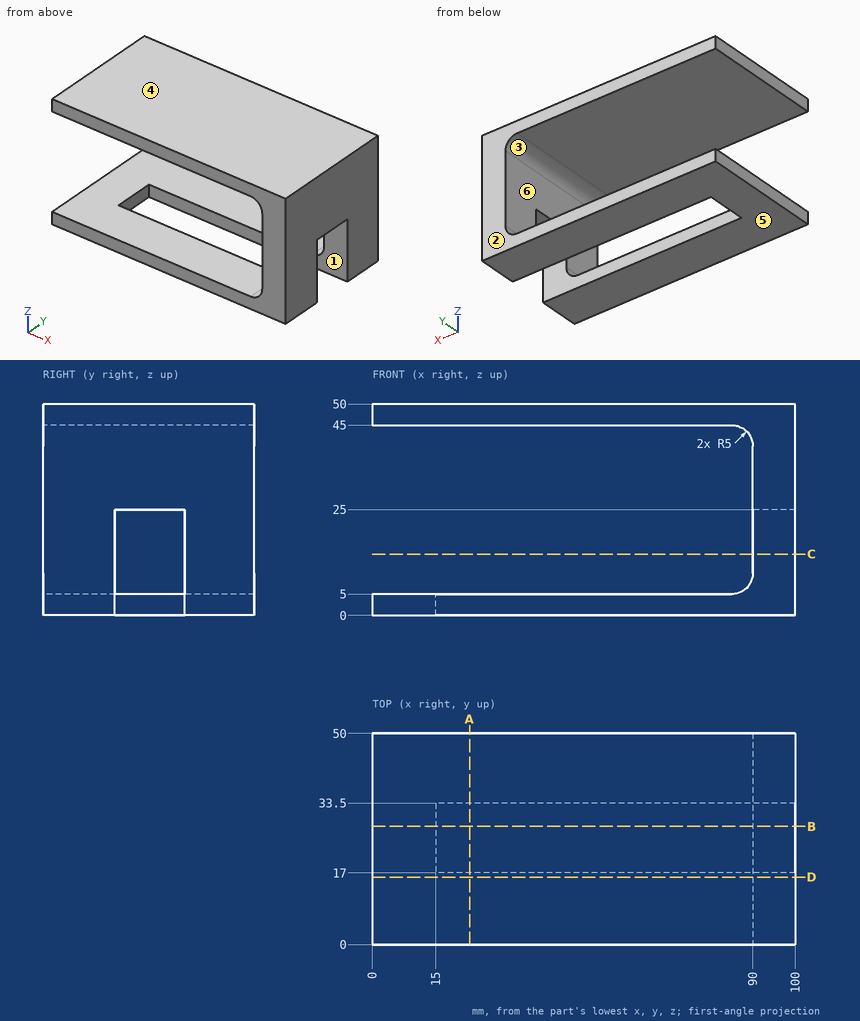
Geometry check sheet. Reference: drawing and pictorial views, mm from the part's lowest x, y, z. A direction names the side the tool comes from. Coordinates: 2 decimals unless noted, no trailing zeros. Order: outer loops, then holes, each group sorted by start corner. A loop starts at its lowest first (then second) coordinate and runs counter-clockwise, first axis right, second up. Notation, with made-up numbers: (12.5, 23) - (68.5, 23) arc R19 ccw to (68.5, 46) - close; hole circle Ø2 at (-11, -39.75). An arc over 180 degrees is marked (long way). One line per item, written item: value.
(1) Thickness scan on probe 1 along Z at (x, y) = (9, 40); probe 2 along Y at (x, z) = (32.5, 2); probe 3 along X at (y, z) = (11, 21). Record the ranges inside material, lowest first. Write a range as from..to.
Data:
probe 1: z = 0..5, 45..50
probe 2: y = 0..17, 33.5..50
probe 3: x = 90..100
(2) Sectioned sample at C-C (z = 14.5). Enter the section's corners in (x, y), and give its area (3 significant figures).
Data:
outline: (90, 0) - (100, 0) - (100, 17) - (90, 17) - close; (90, 33.5) - (100, 33.5) - (100, 50) - (90, 50) - close
area: 335 mm^2
(3) Sectioned sample at D-D (y = 16). Enter the section's corners in (x, z), and give its area (3 significant figures).
Data:
outline: (0, 0) - (100, 0) - (100, 50) - (0, 50) - (0, 45) - (85, 45) arc R5 cw to (90, 40) - (90, 10) arc R5 cw to (85, 5) - (0, 5) - close
area: 1,410 mm^2
(4) Sectioned sample at A-A (x = 23). Enter the section's corners in (y, z), and give its area (4 significant figures).
Data:
outline: (0, 0) - (17, 0) - (17, 5) - (0, 5) - close; (0, 45) - (50, 45) - (50, 50) - (0, 50) - close; (33.5, 0) - (50, 0) - (50, 5) - (33.5, 5) - close
area: 417.5 mm^2
(5) Sectioned sample at B-B (y = 28). Enter the section's corners in (x, z), and give its area (3 significant figures).
Data:
outline: (0, 0) - (15, 0) - (15, 5) - (0, 5) - close; (0, 45) - (85, 45) arc R5 cw to (90, 40) - (90, 25) - (100, 25) - (100, 50) - (0, 50) - close
area: 780 mm^2
(6) Access from +Z, -Z, +X, -X, +Y, -Y to the whole of each face (thin tool, end or side, straight path). Record for the marked faces 1, 2 and 3.
Data:
face 1: -Z, +X
face 2: +Z, -Z, +X, -X, +Y
face 3: -X, +Y, -Y
(7) Depth check by flat-ended pin: pin 1 Ø8 at (y, z) = (27.5, 12.5) entering from -X; pin 2 Ø4 at (y, z) = (25, 2.5) entering from +X; pin 3 Ø3 at (x, y) = (95, 23) entering from -Z; pin 4 Ø3 at (x, y) = (71, 24) entering from -Z. Enter the tip coordinate at first touch or a pass-through.
Data:
pin 1: passes through
pin 2: stops at x = 15
pin 3: stops at z = 25
pin 4: stops at z = 45
(8) Release check for a two-part mould opening along Z. For the marked faces 4, 5 and 6 record: +Z half, -Z half, draft (parallel to the pull), parting line (faces both ways), or undercut.
Data:
face 4: +Z half
face 5: -Z half
face 6: undercut
